Design review of the part shown in the three views and the two pictorial views. Dimensions are in mm from the part's minimum x, y and z. A direction names the side the tool comes from. Give positions to 0.01 mm unless a question says otherwise; leave off trailing zeros. Write each loop counter-clockwise with the first axis right and the second up, starting at its lowest first coordinate (ties: lowest second). Pieces come first, ordered by that corner, then holes.
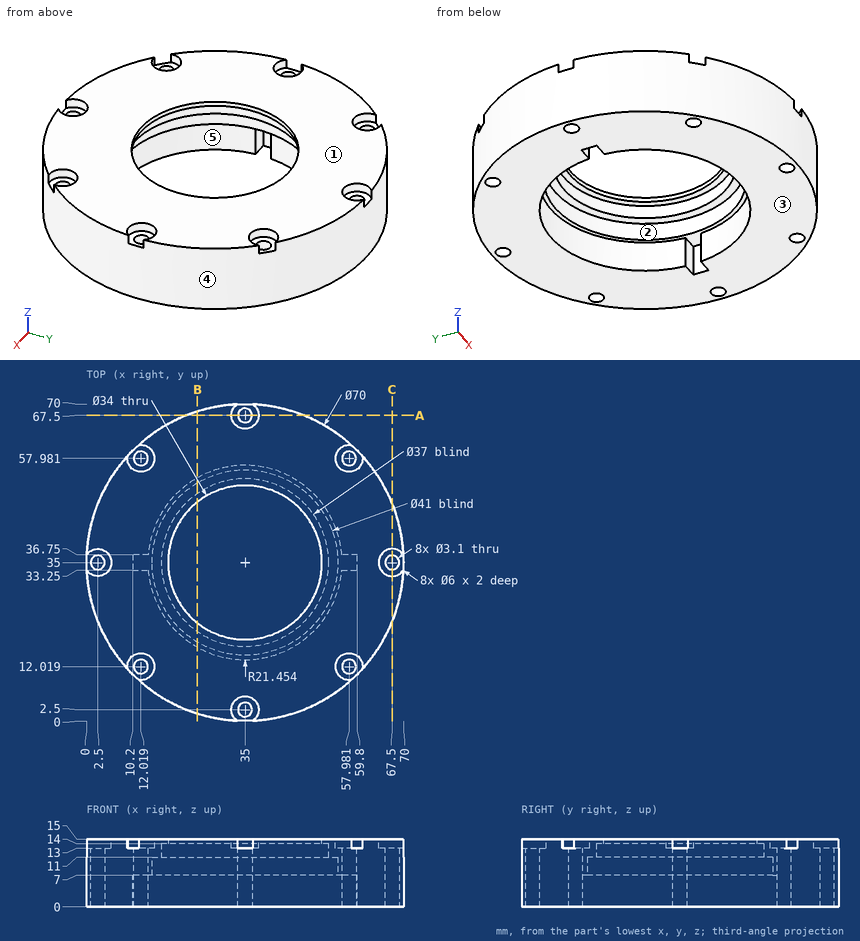
(1) To check wall thickness, follow L1, parallel to Y at x = 35, z = 8.05; L2, parallel to X at y = 26, z = 9.5; L3, parallel to Z at x = 26, y = 52.5. State the ranges of each line that lie inside material, in increasing order.
Resolved:
L1: y = 0 to 0.95, 4.05 to 14.5, 55.5 to 65.95, 69.05 to 70
L2: x = 1.18 to 16.58, 53.42 to 68.82
L3: z = 11 to 15
(2) Mouldability with a two-part tool opening along Y and no side actions: class the marked faces 3, 4 and 5 as pulls with the +Y half, pulls with the -Y half, needs draft (parallel to the pull), parting line crosses it, or undercut.
Resolved:
face 3: needs draft
face 4: parting line crosses it
face 5: undercut
(3) Clearance check with flat-ended pins moving along their axes: P1, Ø4, axis at y = 21.5, z = 3, coming from the +X side; P2, Ø3, axis at x = 11.5, y = 12.5, coming from the +Z side; P3, Ø2.5, axis at x = 58, z = 3.5, coming from the -Y side; P4, Ø3, axis at x = 38.5, y = 48.5, coming from the -Z side. State where each tip first meets the part, or that it passes through.
Resolved:
P1: stops at x = 68.06
P2: stops at z = 13
P3: stops at y = 7.58
P4: passes through
(4) Consider section A-A, the plane y = 67.5. Give the boundary of the cut face in (x, z), then the cut area to 3 significant figures.
Resolved:
outline: (22.01, 0) - (33.45, 0) - (33.45, 13) - (32, 13) - (32, 15) - (22.01, 15) - close; (36.55, 0) - (47.99, 0) - (47.99, 15) - (38, 15) - (38, 13) - (36.55, 13) - close
area: 337 mm2
(5) Consider section B-B, the plane x = 24.5. Give the boundary of the cut face in (y, z), then the cut area to 3 significant figures.
Resolved:
outline: (1.61, 0) - (16.29, 0) - (16.29, 7) - (17.39, 7) - (17.39, 11) - (19.77, 11) - (19.77, 14) - (21.63, 14) - (21.63, 15) - (1.61, 15) - close; (48.37, 14) - (50.23, 14) - (50.23, 11) - (52.61, 11) - (52.61, 7) - (53.71, 7) - (53.71, 0) - (68.39, 0) - (68.39, 15) - (48.37, 15) - close
area: 481 mm2
(6) Tool access review of the marked faces 1 and 2: name each direction out of +Z, -Z, +X, -X, +Y, -Y from which nothing blocks a thin tool from reaching the whole face with its end or side.
Resolved:
face 1: +Z, +X, -X, +Y, -Y
face 2: -Z
